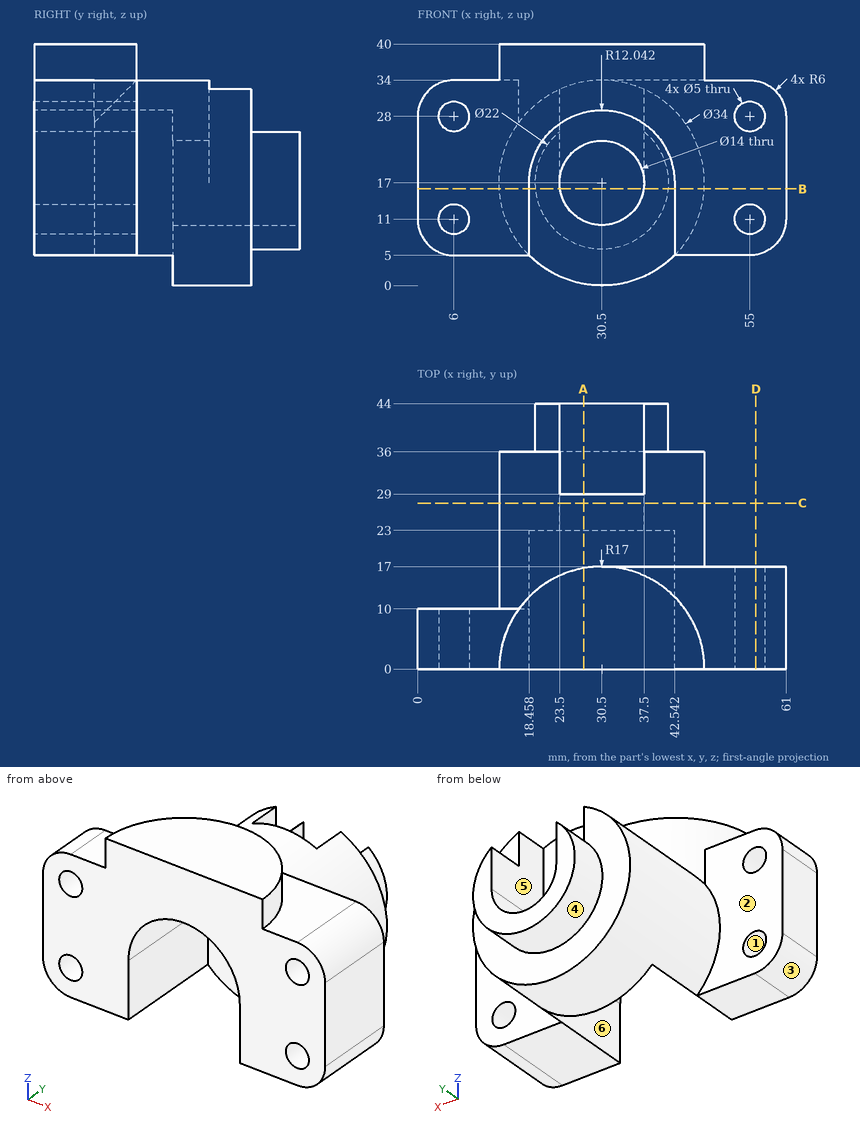
Check sheet for the drawn part. Datum: minimum x, y, z corner. Units: mm. A direction names the side the tool comes from. Give positions to 0.01 mm unless a question says otherwise; leave off trailing zeros. Loops run counter-clockwise (first coordinate to the right, second up) from the corner with the lowest first, then second, coordinate; pieces in that order, holes last.
1) Depth check by flat-ended pin: pin 1 Ø6.5 at (x, z) = (6, 11) entering from +Y; pin 2 Ø22.5 at (x, z) = (30.5, 17) entering from -Y; pin 3 Ø8 at (x, y) = (11.5, 6) entering from -Z; pin 4 Ø4.5 at (x, z) = (55, 11) entering from -Y. Enter the tip coordinate at first touch or a pass-through.
2) Sectioned sample at B-B, the plane z = 16. Enter the section's corners in (x, y) (1 decimal).
3) Sectioned sample at C-C, the plane y = 27.5. Enter the section's corners in (x, z), then the cut area to 3 significant figures.
4) Set-up check for the marked faces 4, 5 and 6: record each of +Z, -Z, +X, -X, +Y, -Y from which the full face is reachable in a straight line by a thin tool's end or side.
5) Thickness scan on line 1 along X through (y, z) = (36.75, 17); line 2 along X through (y, z) = (3.25, 11); line 3 along Z through (x, y) = (51.5, 5.5). Record the ranges inside material, lowest first.
6) Sectioned sample at A-A, the plane x = 27.5. Enter the section's corners in (y, z) (1 decimal).
7) Sectioned sample at D-D, the plane x = 56. Enter the section's corners in (y, z), then the cut area to 3 significant figures.
8) Draft check along Z on the marked faces 1, 2 and 3. Enter one of: pulls with the +Z half, pulls with the -Z half, needs draft (parallel to the pull), parting line crosses it, or undercut.
Answers:
1. pin 1: stops at y = 10
1. pin 2: stops at y = 23
1. pin 3: stops at z = 5
1. pin 4: passes through
2. outline: (0, 0) - (18.5, 0) - (18.5, 23) - (23.6, 23) - (23.6, 44) - (19.5, 44) - (19.5, 36) - (13.5, 36) - (13.5, 10) - (0, 10) - close; (37.4, 23) - (42.5, 23) - (42.5, 0) - (61, 0) - (61, 17) - (47.5, 17) - (47.5, 36) - (41.5, 36) - (41.5, 44) - (37.4, 44) - close
3. outline: circle Ø34 at (30.5, 17); hole circle Ø14 at (30.5, 17)
3. area: 754 mm2
4. face 4: +Y
4. face 5: +Z, +Y
4. face 6: -Z, -Y
5. line 1: x = 19.5 to 23.5, 37.5 to 41.5
5. line 2: x = 0 to 3.5, 8.5 to 18.46, 42.54 to 52.5, 57.5 to 61
5. line 3: z = 5 to 34
6. outline: (0, 28.7) - (23, 28.7) - (23, 23.3) - (29, 23.3) - (29, 33.7) - (16.7, 33.7) - (16.7, 40) - (0, 40) - close; (23, 0.3) - (36, 0.3) - (36, 6.4) - (44, 6.4) - (44, 10.7) - (23, 10.7) - close
7. outline: (0, 5.08) - (17, 5.08) - (17, 8.71) - (0, 8.71) - close; (0, 13.29) - (17, 13.29) - (17, 25.71) - (0, 25.71) - close; (0, 30.29) - (17, 30.29) - (17, 33.92) - (0, 33.92) - close
7. area: 334 mm2
8. face 1: undercut
8. face 2: needs draft
8. face 3: pulls with the -Z half
